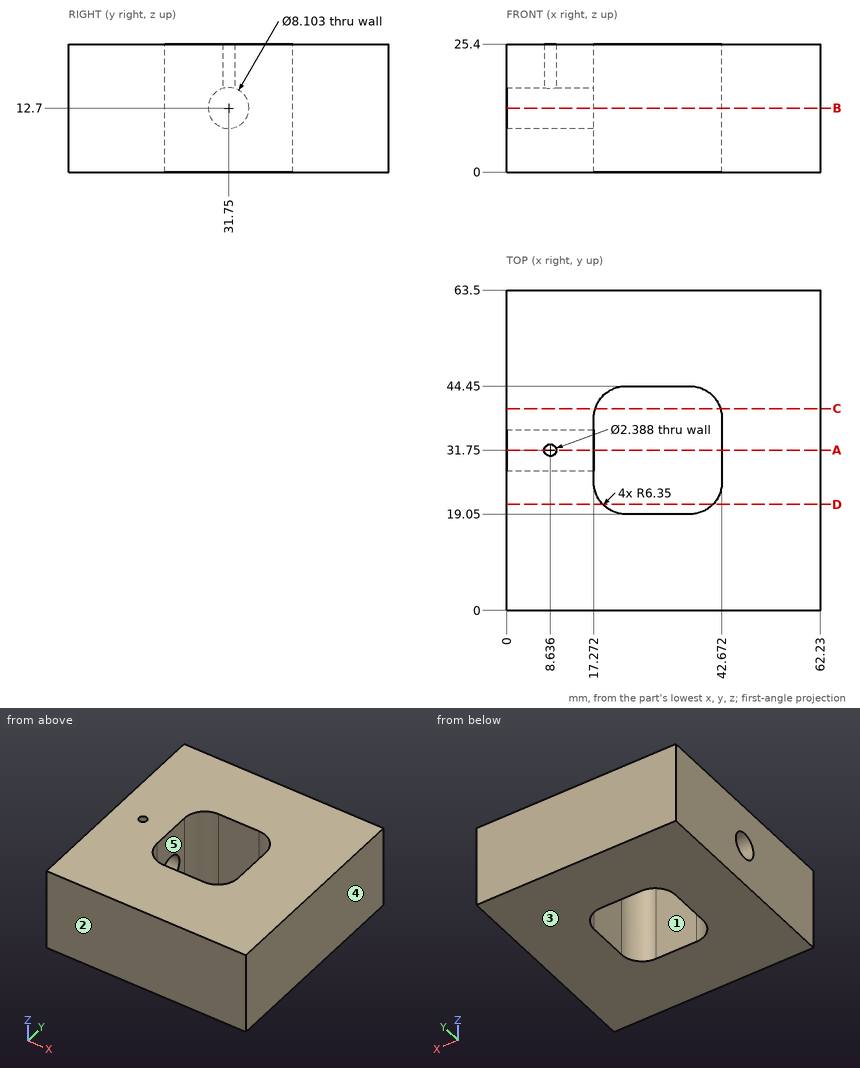
Input: dimensioned drawing with shaded views. Units: mm. Origin: part minimum x, y, z. A direction names the side the tool comes from. Give positions to 0.01 mm unless a question says otherwise; leave off trailing zeros. Order: outer loops, then holes, each group sorted by start corner. A loop starts at its lowest first (then second) coordinate and runs counter-clockwise, first axis right, second up. Notation, with made-up numbers: (56, 3) -> (84, 3) arc R11 ccw to (84, 23) -> close; hole circle Ø3 at (46, -39.75). An arc over 180 degrees is marked (long way). Use one line per item in the form item = value.
1) Section A-A, the plane y = 31.75. Return loops of the section in (x, z), and give its area (3 significant figures).
Response values:
outline = (0, 0) -> (17.27, 0) -> (17.27, 8.65) -> (0, 8.65) -> close; (0, 16.75) -> (7.44, 16.75) -> (7.44, 25.4) -> (0, 25.4) -> close; (9.83, 16.75) -> (17.27, 16.75) -> (17.27, 25.4) -> (9.83, 25.4) -> close; (42.67, 0) -> (62.23, 0) -> (62.23, 25.4) -> (42.67, 25.4) -> close
area = 775 mm^2
2) Section C-C, the plane y = 40. Return loops of the section in (x, z), and give its area (3 significant figures).
Response values:
outline = (0, 0) -> (17.56, 0) -> (17.56, 25.4) -> (0, 25.4) -> close; (42.38, 0) -> (62.23, 0) -> (62.23, 25.4) -> (42.38, 25.4) -> close
area = 950 mm^2
3) Section D-D, the plane y = 21. Return loops of the section in (x, z).
Response values:
outline = (0, 0) -> (19.04, 0) -> (19.04, 25.4) -> (0, 25.4) -> close; (40.9, 0) -> (62.23, 0) -> (62.23, 25.4) -> (40.9, 25.4) -> close
4) Line query: probe 1 along X at (y, z) = (31.75, 23.5); probe 2 along X at (y, z) = (38, 3.5); probe 3 along Y at (x, z) = (34, 20.75). Output: solid intervals per line, ascending.
Response values:
probe_1 = 0 to 7.44, 9.83 to 17.27, 42.67 to 62.23
probe_2 = 0 to 17.27, 42.67 to 62.23
probe_3 = 0 to 19.05, 44.45 to 63.5
5) Section B-B, the plane z = 12.7. Return loops of the section in (x, y).
Response values:
outline = (0, 0) -> (62.23, 0) -> (62.23, 63.5) -> (0, 63.5) -> (0, 35.8) -> (17.27, 35.8) -> (17.27, 38.1) arc R6.35 cw to (23.62, 44.45) -> (36.32, 44.45) arc R6.35 cw to (42.67, 38.1) -> (42.67, 25.4) arc R6.35 cw to (36.32, 19.05) -> (23.62, 19.05) arc R6.35 cw to (17.27, 25.4) -> (17.27, 27.7) -> (0, 27.7) -> close
6) Mould query, pull axis X, two halves, no side actions, for the marked faces 3, 4 and 5. Classes: pulls with the +X half, pulls with the -X half, needs draft (parallel to the pull), parting line crosses it, or undercut.
Response values:
face_3 = needs draft
face_4 = pulls with the +X half
face_5 = undercut
7) Reachability of the marked faces 1 and 2 from +Z, -Z, +X, -X, +Y, -Y: full face, straight path, thin tool, end or side. Return the list, or none.
Response values:
face_1 = +Z, -Z
face_2 = +Z, -Z, +X, -X, -Y
